from build123d import *

# Parameters (mm, degrees)
BOSS_EXTRUDE1_DEPTH = 35
SKETCH2_R           = 2.25
CUT_EXTRUDE1_DEPTH  = 10
CUT_EXTRUDE2_DEPTH  = 5


with BuildPart() as part:
    # Sketch1 → Boss-Extrude1 (new body)
    with BuildSketch(Plane.XY):
        Polygon((8.5, 5), (8.5, 0), (-26.5, 0), (-26.5, -5), (26.5, -5), (26.5, 5), align=None)
    extrude(amount=BOSS_EXTRUDE1_DEPTH)

    # Sketch2 → Cut-Extrude1 (cut)
    with BuildSketch(Plane(origin=(26.5, 0, 0), x_dir=(0, 0, -1), z_dir=(1, 0, 0))):
        with Locations((-22.5, 0)):
            Circle(SKETCH2_R)
        with Locations((-12.5, 0)):
            Circle(SKETCH2_R)
    extrude(amount=-CUT_EXTRUDE1_DEPTH, mode=Mode.SUBTRACT)

    # Sketch3 → Cut-Extrude2 (cut)
    with BuildSketch(Plane(origin=(0, 0, 0), x_dir=(1, 0, 0), z_dir=(0, 1, 0))):
        with BuildLine():
            Line((-22.5, -7.55), (-18.5, -7.55))
            ThreePointArc((-18.5, -7.55), (-16.95, -6), (-18.5, -4.45))
            Line((-18.5, -4.45), (-22.5, -4.45))
            ThreePointArc((-22.5, -4.45), (-24.05, -6), (-22.5, -7.55))
        make_face()
        with BuildLine():
            Line((-22.5, -30.55), (-18.5, -30.55))
            ThreePointArc((-18.5, -30.55), (-16.95, -29), (-18.5, -27.45))
            Line((-18.5, -27.45), (-22.5, -27.45))
            ThreePointArc((-22.5, -27.45), (-24.05, -29), (-22.5, -30.55))
        make_face()
        with BuildLine():
            Line((4.5, -4.45), (0.5, -4.45))
            ThreePointArc((0.5, -4.45), (-1.05, -6), (0.5, -7.55))
            Line((0.5, -7.55), (4.5, -7.55))
            ThreePointArc((4.5, -7.55), (6.05, -6), (4.5, -4.45))
        make_face()
        with BuildLine():
            Line((4.5, -27.45), (0.5, -27.45))
            ThreePointArc((0.5, -27.45), (-1.05, -29), (0.5, -30.55))
            Line((0.5, -30.55), (4.5, -30.55))
            ThreePointArc((4.5, -30.55), (6.05, -29), (4.5, -27.45))
        make_face()
    extrude(amount=-CUT_EXTRUDE2_DEPTH, mode=Mode.SUBTRACT)


solid = part.part
Design review of the part built by this model. Coordinates are the model's own, in mm. A direction names the side the tool comes from. Round coordinates to 2 decimals unless told otherwise and drop trailing zeros. Write each loop counter-clockwise with the first axis right and the second up, starting at its lowest first coordinate (ties: lowest second). Pieces come first, ordered by that corner, then holes. Notation, with made-up numbers: (-39, 59.5) -> (-8, 59.5) arc R23 cw to (-8, 85.5) -> close; hole circle Ø8 at (71, 28.25). An arc over 180 degrees is marked (long way). One line per question, with ' | ' between items.
(1) Take a section at D-D, the plane z = 22.5. State the section outline as (x, y) points.
Result sheet:
outline: (-26.5, -5) -> (26.5, -5) -> (26.5, -2.25) -> (16.5, -2.25) -> (16.5, 2.25) -> (26.5, 2.25) -> (26.5, 5) -> (8.5, 5) -> (8.5, 0) -> (-26.5, 0) -> close
(2) Insertion check: P1, Ø2.5, axis at y = 3, z = 9.5, coming from the -X side; P2, Ø2.5, axis at y = 0, z = 22.5, coming from the +X side; P3, Ø10, axis at x = 2.5, z = 10, coming from the +Y side. Each pin has a flat end and moves straight along its axis. Give the tip position at first contact, or say it passes through.
Result sheet:
P1: x = 8.5 | P2: x = 16.5 | P3: y = 0
(3) Wall thickness on line 1 (X direction, y = -1.5, z = 5); line 2 (Y direction, x = 24.25, z = 12.5); line 3 (Y direction, x = -8, z = 9.5): over which ranges is each line inside the solid? List them lowest first. Write a range as [from, to].
Result sheet:
line 1: [-26.5, -23.68], [-17.32, -0.68], [5.68, 26.5] | line 2: [-5, -2.25], [2.25, 5] | line 3: [-5, 0]
(4) Draft analysis for pull direction Z (two halves, no side actions). For faces 5 (the cylindrical face through (6.05, -2.46, 6.03)), 6 (the flat face through (6, -1, 35)), 7 (the cylindrical face through (6.05, -2.46, 29.03)), 8 (the flat face through (26.5, 0, 17)), state which applies: released by +Z, released by -Z, zero draft, split by the parting line, or undercut.
Result sheet:
face 5: undercut | face 6: released by +Z | face 7: undercut | face 8: zero draft
(5) Machinability: for faces 1 (the flat face through (-9, 0, 17)), 2 (the flat face through (3, -2, 4.45)), 3 (the flat face through (16.5, 0, 23)), 4 (the flat face through (6, -1, 0)), which of the approach directions +Z, -Z, +X, -X, +Y, -Y give a long, thin tool a straight path to every point of the face, cutting with its end or side? Answer none if there is none.
Result sheet:
face 1: +Z, -Z, -X, +Y | face 2: +Y, -Y | face 3: +X | face 4: -Z, +X, -X, +Y, -Y
(6) Take a section at C-C, the plane y = -3. State the section outline as (x, z) points.
Result sheet:
outline: (-26.5, 0) -> (26.5, 0) -> (26.5, 35) -> (-26.5, 35) -> close; hole (-22.5, 4.45) -> (-18.5, 4.45) arc R1.55 ccw to (-18.5, 7.55) -> (-22.5, 7.55) arc R1.55 ccw to start; hole (-22.5, 27.45) -> (-18.5, 27.45) arc R1.55 ccw to (-18.5, 30.55) -> (-22.5, 30.55) arc R1.55 ccw to start; hole (0.5, 4.45) -> (4.5, 4.45) arc R1.55 ccw to (4.5, 7.55) -> (0.5, 7.55) arc R1.55 ccw to start; hole (0.5, 27.45) -> (4.5, 27.45) arc R1.55 ccw to (4.5, 30.55) -> (0.5, 30.55) arc R1.55 ccw to start
(7) Take a section at B-B, the plane x = 19. State the section outline as (y, z) points.
Result sheet:
outline: (-5, 0) -> (5, 0) -> (5, 35) -> (-5, 35) -> close; hole circle Ø4.5 at (0, 12.5); hole circle Ø4.5 at (0, 22.5)
(8) Take a section at A-A, the plane z = 29. State the section outline as (x, y) points, and give its area (3 significant figures).
Result sheet:
outline: (-26.5, -5) -> (-24.05, -5) -> (-24.05, 0) -> (-26.5, 0) -> close; (-16.95, -5) -> (-1.05, -5) -> (-1.05, 0) -> (-16.95, 0) -> close; (6.05, -5) -> (26.5, -5) -> (26.5, 5) -> (8.5, 5) -> (8.5, 0) -> (6.05, 0) -> close | area: 284 mm2
